from build123d import *

# Parameters (mm, degrees)
ESQUISSE1_W        = 12
ESQUISSE1_H        = 12.5
BOSS_EXTRU_1_DEPTH = 9.5
ESQUISSE3_R        = 3.1
BOSS_EXTRU_2_DEPTH = 7.5
ESQUISSE4_R        = 1.5
BOSS_EXTRU_3_DEPTH = 15
CONG_3_R           = 1


with BuildPart() as part:
    # Esquisse1 → Boss.-Extru.1 (new body)
    with BuildSketch(Plane.XY):
        with Locations((-57.806805708, 22.931818182)):
            Rectangle(ESQUISSE1_W, ESQUISSE1_H)
    extrude(amount=BOSS_EXTRU_1_DEPTH)

    # Esquisse3 → Boss.-Extru.2 (add)
    with BuildSketch(Plane.XY.offset(9.5)):
        with Locations((-57.806805708, 22.931818182)):
            Circle(ESQUISSE3_R)
    extrude(amount=BOSS_EXTRU_2_DEPTH)

    # Esquisse4 → Boss.-Extru.3 (add)
    with BuildSketch(Plane.XY.offset(17)):
        with Locations((-57.806805708, 22.931818182)):
            Circle(ESQUISSE4_R)
    extrude(amount=BOSS_EXTRU_3_DEPTH)

    # Congé3
    cong_3_edges = [part.edges().sort_by_distance(p)[0] for p in [
        (-59.306805708, 22.931818182, 17),
        (-59.306805708, 22.931818182, 32),
    ]]
    fillet(cong_3_edges, radius=CONG_3_R)


solid = part.part
The listing builds one solid part. Answer for the finished solid, in the listing's coordinates (mm). A direction names the side the tool comes from. Round coordinates to 2 decimals unless told otherwise and drop trailing zeros. Order: outer loops, then holes, each group sorted by start corner. A loop starts at its lowest first (then second) coordinate and runs counter-clockwise, first axis right, second up. Notation, with made-up numbers: (-2, -7) -> (31, -7) arc R27 ccw to (31, 15) -> close; hole circle Ø3 at (31, 24.5). An arc over 180 degrees is marked (long way). One line per item, written item: value.
Item 1: Find section D-D, the plane x = -53.5. Give the vertices of the cut face in (y, z).
Taken from the geometry:
outline: (16.68, 0) -> (29.18, 0) -> (29.18, 9.5) -> (16.68, 9.5) -> close
Item 2: Find section C-C, the plane z = 16.5. Give the vertices of the cut face in (x, y).
Taken from the geometry:
outline: circle Ø6.2 at (-57.81, 22.93)
Item 3: Straight lines are drawn through the part: L1, parallel to Z at x = -54, y = 28.75; L2, parallel to X at y = 22.75, z = 16.5; L3, parallel to Z at x = -60.75, y = 23.75. For each, find the intervals that lie inside material, in ascending order.
Taken from the geometry:
L1: z = 0 to 9.5
L2: x = -60.9 to -54.71
L3: z = 0 to 17
Item 4: Find section A-A, the plane x = -55. Give the vertices of the cut face in (y, z), then the cut area to 3 significant figures.
Taken from the geometry:
outline: (16.68, 0) -> (29.18, 0) -> (29.18, 9.5) -> (24.25, 9.5) -> (24.25, 17) -> (21.62, 17) -> (21.62, 9.5) -> (16.68, 9.5) -> close
area: 138 mm2
Item 5: Find section B-B, the plane y = 28.75. Give the vertices of the cut face in (x, z).
Taken from the geometry:
outline: (-63.81, 0) -> (-51.81, 0) -> (-51.81, 9.5) -> (-63.81, 9.5) -> close
Item 6: Given P1, Ø4, axis at x = -55, z = 16.5, coming from the -Y side; P2, Ø2, axis at y = 18, z = 13.5, coming from the -X side (3 decimals); P3, Ø1.5, axis at x = -59, y = 21.5, coming from the +Z side; P4, Ø6, axis at y = 24, z = 17.5, coming from the +X side, each flat-ended and moving along its own axis, determine where each tip first touches the part or whether it passes through.
Taken from the geometry:
P1: stops at y = 19.94
P2: passes through
P3: stops at z = 31.79
P4: stops at x = -54.71
Item 7: For faces 1 (the flat face through (-58, 29.182, 5)), 2 (the flat face through (-55, 23, 17)), determine the directions among +Z, -Z, +X, -X, +Y, -Y from which every point of the face is accessible in a straight line to the end or side of a thin tool.
Taken from the geometry:
face 1: +Z, -Z, +X, -X, +Y
face 2: +Z
